CAD build for the part. Positions are in the model's coordinates, mm. A direction names the side the tool comes from. Round coordinates to 2 decimals unless told otherwise and drop trailing zeros. Loops run counter-clockwise (first coordinate to the right, second up) from the corner with the lowest first, then second, coordinate; pieces in that order, holes last. Notation, with made-up numbers: (22, -11) - (50, -11) arc R8 cw to (50, -3) - close; hole circle Ø3 at (15, 12.25). An arc over 180 degrees is marked (long way). Use one line per item in the form item = value.
from build123d import *

# Parameters (mm, degrees)
F1_DEPTH  = 25.4
F1_FACE_W = 50.8
F1_FACE_H = 50.8
F2_DEPTH  = 25.4
F3_R      = 6.35
F4_DEPTH  = 5.08
F6_DEPTH  = 5.08
F8_DEPTH  = 5.08
F9_DEPTH  = 6.35


with BuildPart() as f1:
    # F0 (on Front) → F1 (new body)
    with BuildSketch(Plane.XZ):
        Polygon((-25.4, 25.4), (-25.4, 0), (-25.4, -25.4), (25.4, -25.4), (25.4, 25.4), align=None)
    extrude(amount=F1_DEPTH)

    # F1_face (on face) → F2 (join)
    with BuildSketch(Plane(origin=(0, 0, 0), x_dir=(1, 0, 0), z_dir=(0, 1, 0))):
        Rectangle(F1_FACE_W, F1_FACE_H)
    extrude(amount=F2_DEPTH)

    # F3 (on face) → F4 (cut)
    with BuildSketch(Plane.XY.offset(25.4)):
        Circle(F3_R)
    extrude(amount=-F4_DEPTH, mode=Mode.SUBTRACT)

    # F5 (on face) → F6 (cut)
    with BuildSketch(Plane(origin=(0, 25.4, 0), x_dir=(-1, 0, 0), z_dir=(0, 1, 0))):
        with BuildLine():
            Line((-12.7, 0), (0, 0))
            Line((0, 0), (12.7, 0))
            Line((12.7, 0), (25.4, 0))
            Line((25.4, 0), (25.4, 25.4))
            Line((25.4, 25.4), (-12.7, 25.4))
            Line((-12.7, 25.4), (-12.7, 19.05))
            ThreePointArc((-12.7, 19.05), (-8.209872, 17.190128), (-6.35, 12.7))
            ThreePointArc((-6.35, 12.7), (-8.209872, 8.209872), (-12.7, 6.35))
            Line((-12.7, 6.35), (-12.7, 0))
        make_face()
        with BuildLine():
            Line((-25.4, 0), (-12.7, 0))
            Line((-12.7, 0), (-12.7, 6.35))
            ThreePointArc((-12.7, 6.35), (-19.05, 12.7), (-12.7, 19.05))
            Line((-12.7, 19.05), (-12.7, 25.4))
            Line((-12.7, 25.4), (-25.4, 25.4))
            Line((-25.4, 25.4), (-25.4, 0))
        make_face()
        with BuildLine():
            Line((25.4, 0), (12.7, 0))
            Line((12.7, 0), (12.7, -6.23736))
            ThreePointArc((12.7, -6.23736), (17.269776, -8.130224), (19.16264, -12.7))
            ThreePointArc((19.16264, -12.7), (17.269776, -17.269776), (12.7, -19.16264))
            Line((12.7, -19.16264), (12.7, -25.4))
            Line((12.7, -25.4), (25.4, -25.4))
            Line((25.4, -25.4), (25.4, 0))
        make_face()
        with BuildLine():
            Line((12.7, 0), (0, 0))
            Line((0, 0), (-12.7, 0))
            Line((-12.7, 0), (-25.4, 0))
            Line((-25.4, 0), (-25.4, -25.4))
            Line((-25.4, -25.4), (12.7, -25.4))
            Line((12.7, -25.4), (12.7, -19.16264))
            ThreePointArc((12.7, -19.16264), (6.23736, -12.7), (12.7, -6.23736))
            Line((12.7, -6.23736), (12.7, 0))
        make_face()
    extrude(amount=-F6_DEPTH, mode=Mode.SUBTRACT)

    # F7 (on face) → F8 (cut)
    with BuildSketch(Plane(origin=(0, 0, -25.4), x_dir=(1, 0, 0), z_dir=(0, 0, -1))):
        with BuildLine():
            Line((-12.7, -12.7), (-12.7, -6.35))
            ThreePointArc((-12.7, -6.35), (-19.05, -12.7), (-12.7, -19.05))
            Line((-12.7, -19.05), (-12.7, -12.7))
        make_face()
        with BuildLine():
            ThreePointArc((-6.35, -12.7), (-8.209872, -8.209872), (-12.7, -6.35))
            Line((-12.7, -6.35), (-12.7, -12.7))
            Line((-12.7, -12.7), (-12.7, -19.05))
            ThreePointArc((-12.7, -19.05), (-8.209872, -17.190128), (-6.35, -12.7))
        make_face()
        with BuildLine():
            Line((6.35, 0), (0, 0))
            Line((0, 0), (-6.35, 0))
            ThreePointArc((-6.35, 0), (0, -6.35), (6.35, 0))
        make_face()
        with BuildLine():
            Line((-6.35, 0), (0, 0))
            Line((0, 0), (6.35, 0))
            ThreePointArc((6.35, 0), (0, 6.35), (-6.35, 0))
        make_face()
        with BuildLine():
            Line((12.7, 12.7), (12.7, 6.35))
            ThreePointArc((12.7, 6.35), (17.190128, 8.209872), (19.05, 12.7))
            ThreePointArc((19.05, 12.7), (17.190128, 17.190128), (12.7, 19.05))
            Line((12.7, 19.05), (12.7, 12.7))
        make_face()
        with BuildLine():
            ThreePointArc((12.7, 19.05), (6.35, 12.7), (12.7, 6.35))
            Line((12.7, 6.35), (12.7, 12.7))
            Line((12.7, 12.7), (12.7, 19.05))
        make_face()
    extrude(amount=-F8_DEPTH, mode=Mode.SUBTRACT)

    # F5 (on face) → F9 (join)
    with BuildSketch(Plane(origin=(0, 25.4, 0), x_dir=(-1, 0, 0), z_dir=(0, 1, 0))):
        with BuildLine():
            Line((-12.7, 0), (0, 0))
            Line((0, 0), (12.7, 0))
            Line((12.7, 0), (25.4, 0))
            Line((25.4, 0), (25.4, 25.4))
            Line((25.4, 25.4), (-12.7, 25.4))
            Line((-12.7, 25.4), (-12.7, 19.05))
            ThreePointArc((-12.7, 19.05), (-8.209872, 17.190128), (-6.35, 12.7))
            ThreePointArc((-6.35, 12.7), (-8.209872, 8.209872), (-12.7, 6.35))
            Line((-12.7, 6.35), (-12.7, 0))
        make_face()
        with BuildLine():
            Line((12.7, 0), (0, 0))
            Line((0, 0), (-12.7, 0))
            Line((-12.7, 0), (-25.4, 0))
            Line((-25.4, 0), (-25.4, -25.4))
            Line((-25.4, -25.4), (12.7, -25.4))
            Line((12.7, -25.4), (12.7, -19.16264))
            ThreePointArc((12.7, -19.16264), (6.23736, -12.7), (12.7, -6.23736))
            Line((12.7, -6.23736), (12.7, 0))
        make_face()
        with BuildLine():
            Line((25.4, 0), (12.7, 0))
            Line((12.7, 0), (12.7, -6.23736))
            ThreePointArc((12.7, -6.23736), (17.269776, -8.130224), (19.16264, -12.7))
            ThreePointArc((19.16264, -12.7), (17.269776, -17.269776), (12.7, -19.16264))
            Line((12.7, -19.16264), (12.7, -25.4))
            Line((12.7, -25.4), (25.4, -25.4))
            Line((25.4, -25.4), (25.4, 0))
        make_face()
        with BuildLine():
            Line((-25.4, 0), (-12.7, 0))
            Line((-12.7, 0), (-12.7, 6.35))
            ThreePointArc((-12.7, 6.35), (-19.05, 12.7), (-12.7, 19.05))
            Line((-12.7, 19.05), (-12.7, 25.4))
            Line((-12.7, 25.4), (-25.4, 25.4))
            Line((-25.4, 25.4), (-25.4, 0))
        make_face()
    extrude(amount=-F9_DEPTH)


solid = f1.part
1) Flat gauge pins, fed straight in: pin 1 (6.5 mm diameter, centred on x = 13, y = -12, fed in from -Z); pin 2 (7.5 mm diameter, centred on x = 0, y = 0, fed in from +Z). Where does each tip first touch, or does it go through?
Report:
pin_1 = -20.32
pin_2 = 20.32
2) Slice it at A-A (x = 0). Write the cut outline in (y, z), plus the area to 3 significant figures.
Report:
outline = (-25.4, -25.4) - (-6.35, -25.4) - (-6.35, -20.32) - (6.35, -20.32) - (6.35, -25.4) - (25.4, -25.4) - (25.4, 25.4) - (6.35, 25.4) - (6.35, 20.32) - (-6.35, 20.32) - (-6.35, 25.4) - (-25.4, 25.4) - close
area = 2,450 mm^2
3) Tool access for faces 1 (the flat face through (0, 0, 20.32)), 2 (the cylindrical face through (6.057, -1.907, -22.896)), 3 (the flat face through (25.4, 0, 0)): list every direction of +Z, -Z, +X, -X, +Y, -Y with a clear straight run to the whole face (end or side of a thin tool).
Report:
face_1 = +Z
face_2 = -Z
face_3 = +Z, -Z, +X, +Y, -Y
4) Slice it at D-D (x = -8.5). Write the cut outline in (y, z).
Report:
outline = (-25.4, -25.4) - (7.94, -25.4) - (7.94, -20.32) - (17.46, -20.32) - (17.46, -25.4) - (25.4, -25.4) - (25.4, 25.4) - (-25.4, 25.4) - close
5) Two-plate mould, pull along Y, no slides. Class faces 4 (the flat face through (-25.4, 0, 0)), 5 (the flat face through (0, 0, -20.32)), 6 (the flat face through (0, 25.4, 0)): +Y half, -Y half, draft (parallel to the pull), parting line (faces both ways), or undercut.
Report:
face_4 = draft
face_5 = undercut
face_6 = +Y half
6) Slice it at C-C (y = 10). Write the cut outline in (x, z).
Report:
outline = (-25.4, -25.4) - (-18.45, -25.4) - (-18.45, -20.32) - (-6.95, -20.32) - (-6.95, -25.4) - (25.4, -25.4) - (25.4, 25.4) - (-25.4, 25.4) - close
7) Drill centre lines: probe 1 along Y at (x, z) = (0, 23.8); probe 2 along Z at (x, y) = (-14, 8); probe 3 along Z at (x, y) = (-3, -2). Where is each one in solid material? Low to high.
Report:
probe_1 = -25.4 to -6.35, 6.35 to 25.4
probe_2 = -20.32 to 25.4
probe_3 = -20.32 to 20.32
